Build history of the part. All positions in model axes, mm. Give positions to 0.01 mm unless a question says otherwise; leave off trailing zeros. Loops run counter-clockwise (first coordinate to the right, second up) from the corner with the lowest first, then second, coordinate; pieces in that order, holes last. Notation, with made-up numbers: M 70,46 L 99,46 A12 cw 99,57 Z; hole C 77.5,2.5 d9. An arc over 180 degrees is marked long. Put each result on its own line as item: value.
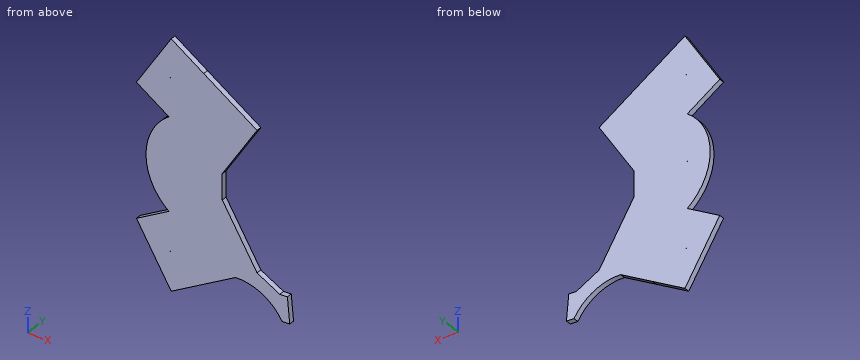
Autodesk Inventor part; units mm, degrees
ref_plane "YZ Plane" through (0, 0, 0) normal (1, 0, 0) x (0, 1, 0)
ref_plane "XZ Plane" through (0, 0, 0) normal (0, 1, 0) x (-1, 0, 0)
ref_plane "XY Plane" through (0, 0, 0) normal (0, 0, 1) x (1, 0, 0)
sketch "Sketch1" plane through (0, 0, 0) normal (0, 1, 0) x (-1, 0, 0)
  line L0 (-21, -5) -> (-21, 5)
  line L1 (0, -18) -> (-21, -5)
  line L2 (0, 18) -> (-21, 5)
  line L3 (-21, -5) -> (-34.6852, -27.1069)
  line L4 (0, -18) -> (-13.6852, -40.1069)
  line L5 (-13.6852, -40.1069) -> (-34.6852, -27.1069)
  line L6 (-21, 5) -> (-34.6852, 27.1069)
  line L7 (0, 18) -> (-13.6852, 40.1069)
  line L8 (-13.6852, 40.1069) -> (-34.6852, 27.1069)
  arc A0 (0, -18) -> (0, 18) centre (-13.5, 0) ccw
  circle A1 centre (0, 0) radius 0.1
  line L9 (-13.6852, -40.1069) -> (0, -18)
  line L10 (0, -18) -> (12.754, -25.8953)
  line L11 (12.754, -25.8953) -> (-0.9312, -48.0022)
  line L12 (-0.9312, -48.0022) -> (-13.6852, -40.1069)
  line L13 (0, 18) -> (-13.6852, 40.1069)
  line L14 (-13.6852, 40.1069) -> (-0.9312, 48.0022)
  line L15 (-0.9312, 48.0022) -> (12.754, 25.8953)
  line L16 (12.754, 25.8953) -> (0, 18)
  line L17 (-34.6852, -27.1069) -> (-43.636, -31.5659)
  line L18 (-44.556, -41.5235) -> (-43.636, -31.5659)
  arc A2 (-26.1826, -32.3704) -> (-44.556, -41.5235) centre (-28.2096, -51.3191) ccw
  line L19 (-26.1826, -32.3704) -> (-34.6852, -27.1069)
  line L20 (-34.6852, -27.1069) -> (-43.636, -31.5659)
  line L21 (-43.636, -31.5659) -> (-44.556, -41.5235)
  arc A3 (-26.1826, -32.3704) -> (-44.556, -41.5235) centre (-28.2096, -51.3191) ccw
  line L22 (-43.636, -31.5659) -> (-46.6233, -31.2899)
  line L23 (-44.556, -41.5235) -> (-47.5433, -41.2475)
  line L24 (-47.5433, -41.2475) -> (-46.6233, -31.2899)
  line L25 (5.9114, -36.9488) -> (-6.8426, -29.0534)
  line L26 (5.9114, 36.9488) -> (-6.8426, 29.0534)
  circle A4 centre (-0.4656, -33.0011) radius 0.1
  circle A5 centre (-0.4656, 33.0011) radius 0.1
  point P0 (-21, 0)
  point P1 (-39.1606, -29.3364)
  dimension "d5" = 10
  dimension "d6" = 26
  dimension "d7" = 26
  dimension "d8" = 26
  dimension "d9" = 26
  dimension "d10" = 36
  dimension "d12" = 0.2
  dimension "d13" = 15
  dimension "d14" = 15
  dimension "d22" = 3
  dimension "d25" = 0.2
  dimension "d26" = 0.2
extrude "Extrusion1" add sketch "Sketch1" along normal blind 2 contours L0 L2 A0 L1 | L1 L4 L5 L3 | L6 L8 L7 L2 | L10 L11 L25 A4 L4 | L7 L26 A5 L15 L16 | L25 A4 L11 L12 L4 | L7 L14 L15 L26 A5 | A4 L25 | L25 A4 | A5 L26 | L26 A5
extrude "Extrusion2" add sketch "Sketch1" along normal blind 2 contours L5 A2 L18 L17
extrude "Extrusion3" add sketch "Sketch1" along normal blind 2 contours L18 L23 L24 L22
extrude "Extrusion4" cut sketch "Sketch1" along normal blind 2 contours A4 L25 | L25 A4 | A5 L26 | L26 A5
properties part number "drzak_buzirka"
Q1. Drop a flat-ended pin along its axis: pin 1 Ø1 at (y, z) = (0.5, -8) entering from -X. Give the stop position or say it passes through.
Here are the results:
pin 1: x = -7.71
Q2. Slice it at C-C (y = 1.65). List the corners of the cut face in (x, z).
Here are the results:
outline: M -12.75,-25.9 L 0.93,-48 L 13.69,-40.11 L 26.18,-32.37 A19.06 cw 44.56,-41.52 L 47.54,-41.25 L 46.62,-31.29 L 43.64,-31.57 L 34.69,-27.11 L 21,-5 L 21,5 L 34.69,27.11 L 13.69,40.11 L 0.93,48 L -12.75,25.9 L 0,18 A22.5 ccw 0,-18 Z; hole C 0,0 d0.2; hole C 0.47,-33 d0.2; hole C 0.47,33 d0.2
Q3. Probe line 1 (Z direction, x = 21.5, y = 1.25); line 2 (X direction, y = 0.25, z = -37.5); line 3 (Z direction, x = 12, y = 1.9). List the from-to ranges inside material, lowest first. Write a range as from..to.
Here are the results:
line 1: -35.27..-5.81, 5.81..35.27
line 2: -5.57..17.9, 41.33..47.2
line 3: -41.15..41.15
Q4. Slice it at B-B (x = 30.5). List the corners of the cut face in (y, z).
Here are the results:
outline: M 0,-32.4 L 2,-32.4 L 2,-20.35 L 0,-20.35 Z; M 0,20.35 L 2,20.35 L 2,29.7 L 0,29.7 Z
Q5. Slice it at D-D (z = 16). List the corners of the cut face in (x, y).
Here are the results:
outline: M -2.32,0 L 27.81,0 L 27.81,2 L -2.32,2 Z
Q6. Slice it at A-A (z = -38). List the corners of the cut face in (x, y).
Here are the results:
outline: M -5.26,0 L 17.09,0 L 17.09,2 L -5.26,2 Z; M 41.84,0 L 47.24,0 L 47.24,2 L 41.84,2 Z
